from build123d import *

# Parameters (mm, degrees)
F0_W     = 25.4
F0_H     = 146.05
F1_DEPTH = 25.4
F3_DEPTH = 19.05
F4_R     = 6.35
F5_DEPTH = 37.689491
F6_R     = 9.525
F7_DEPTH = 25.4


with BuildPart() as f1:
    # F0 (on Top) → F1 (new body)
    with BuildSketch(Plane.XY):
        with Locations((-0.411509, 73.025)):
            Rectangle(F0_W, F0_H)
    extrude(amount=F1_DEPTH)

    # F2 (on Top) → F3 (join)
    with BuildSketch(Plane.XY):
        with BuildLine():
            Line((25.4, 38.1), (0, 38.1))
            Line((0, 38.1), (-25.4, 38.1))
            Line((-25.4, 38.1), (-25.4, -97.86834))
            ThreePointArc((-25.4, -97.86834), (0, -101.6), (25.4, -97.86834))
            Line((25.4, -97.86834), (25.4, 38.1))
        make_face()
    extrude(amount=-F3_DEPTH)

    # F4 (on face) → F5 (cut, through all)
    with BuildSketch(Plane.YZ.offset(12.288491)):
        with Locations((95.25, 12.7)):
            Circle(F4_R)
    extrude(amount=-F5_DEPTH, mode=Mode.SUBTRACT)

    # F6 (on face) → F7 (cut)
    with BuildSketch(Plane.XY):
        with Locations((0, -69.85)):
            Circle(F6_R)
    extrude(amount=-F7_DEPTH, mode=Mode.SUBTRACT)


solid = f1.part
Check sheet for the modelled part. Datum: model origin and axes. Units: mm. A direction names the side the tool comes from. Round coordinates to 2 decimals unless told otherwise and drop trailing zeros. Loops run counter-clockwise (first coordinate to the right, second up) from the corner with the lowest first, then second, coordinate; pieces in that order, holes last. Notation, with made-up numbers: (-31.5, 26) -> (0.5, 26) arc R21 ccw to (0.5, 31) -> close; hole circle Ø11 at (-1, 36.25). An arc over 180 degrees is marked (long way). Put each result on its own line as item: value. Start each with the question number.
1. Section check D-D (z = -6.5). Enter the section's corners in (x, y) (3 decimals), plus the area to 3 significant figures.
2. Section check C-C (y = -69.85). Enter the section's corners in (x, z) (3 decimals), plus the area to 3 significant figures.
3. Section check B-B (z = 12.7). Enter the section's corners in (x, y).
4. Access from +Z, -Z, +X, -X, +Y, -Y to the whole of each face (thin tool, end or side, straight path). Record for faces 1 (the face through (-13.112, 72, 13)), 2 (the face through (-1, 93, 0)), 3 (the face through (-1, 0, 13)), 4 (the face through (12.288, 72, 13)).
5. Gauge pin test, flat ends, axial feed: pin 1 (1.5 mm diameter, centred on y = 111.5, z = 2.5, fed in from +X); pin 2 (10 mm diameter, centred on y = 95.25, z = 12.7, fed in from +X); pin 3 (7.5 mm diameter, centred on x = 2.5, z = 10, fed in from -Y); pin 4 (5 mm diameter, centred on x = -13, z = -9.5, fed in from +Y). Record the tip position at first contact, or that the pin passes through.
6. Section check A-A (x = 0). Enter the section's corners in (y, z) (3 decimals).
7. Scan lines: probe 1 along X at (y, z) = (-69, -5); probe 2 along Y at (x, z) = (0, -6) (3 decimals); probe 3 along Y at (x, z) = (6, 12). Record each from-to range of solid material in increasing order.
8. Draft check along X on faces 5 (the face through (0, -31, -19.05)), 6 (the face through (-25.4, -29, -9)), 7 (the face through (-0.4, -101.6, -9.4)), 8 (the face through (-2.06, -79.15, -9.39)). Enter one of: +X half, -X half, draft (parallel to the pull), parting line (faces both ways), or undercut.
Findings:
1. outline: (-25.4, -97.868) arc R88.31 ccw to (25.4, -97.868) -> (25.4, 38.1) -> (-25.4, 38.1) -> close; hole circle Ø19.05 at (0, -69.85)
1. area: 6,750 mm^2
2. outline: (-25.4, -19.05) -> (-9.525, -19.05) -> (-9.525, 0) -> (-25.4, 0) -> close; (9.525, -19.05) -> (25.4, -19.05) -> (25.4, 0) -> (9.525, 0) -> close
2. area: 605 mm^2
3. outline: (-13.11, 0) -> (12.29, 0) -> (12.29, 88.9) -> (-13.11, 88.9) -> close; (-13.11, 101.6) -> (12.29, 101.6) -> (12.29, 146.05) -> (-13.11, 146.05) -> close
4. face 1: +Z, -X, +Y, -Y
4. face 2: -Z, +X, -X, +Y
4. face 3: +Z, +X, -X, -Y
4. face 4: +Z, +X, +Y, -Y
5. pin 1: stops at x = 12.29
5. pin 2: passes through
5. pin 3: stops at y = 0
5. pin 4: stops at y = 38.1
6. outline: (-101.6, -19.05) -> (-79.375, -19.05) -> (-79.375, 0) -> (-101.6, 0) -> close; (-60.325, -19.05) -> (38.1, -19.05) -> (38.1, 0) -> (146.05, 0) -> (146.05, 25.4) -> (0, 25.4) -> (0, 0) -> (-60.325, 0) -> close; hole circle Ø12.7 at (95.25, 12.7)
7. probe 1: x = -25.4 to -9.49, 9.49 to 25.4
7. probe 2: y = -101.6 to -79.375, -60.325 to 38.1
7. probe 3: y = 0 to 88.94, 101.56 to 146.05
8. face 5: draft
8. face 6: -X half
8. face 7: parting line
8. face 8: undercut
